For this review, take the finished solid that the model builds, in its own axes (mm). Face numbers are marked on the shaded views. A direction names the side the tool comes from. Round coordinates to 2 decimals unless told otherwise and drop trailing zeros. Order: outer loops, then holes, each group sorted by start corner. A loop starts at its lowest first (then second) coordinate and runs counter-clockwise, first axis right, second up. Notation, with made-up numbers: (10.5, -13.75) - (37.5, -13.75) arc R16 cw to (37.5, -6.75) - close; hole circle Ø9 at (18.25, 84). An arc over 180 degrees is marked (long way). One line per question, with ' | ' between items.
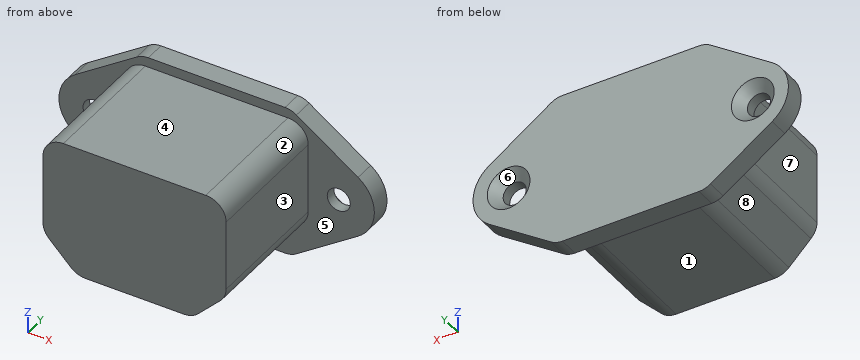
```python
from build123d import *

# Parameters (mm, degrees)
SKIZZE1_W                                    = 27
SKIZZE1_H                                    = 19.5
AUFSATZ_LINEAR_AUSTRAGEN1_DEPTH              = 19.6
FASE1_SIZE                                   = 5
AUFSATZ_LINEAR_AUSTRAGEN2_DEPTH              = 3
VERRUNDUNG1_R                                = 3
FORMSENKUNG_F_R_M3_LINSENSENKSCHRAUB_2_COUNT = 2
FORMSENKUNG_F_R_M3_LINSENSENKSCHRAUB_2_PITCH = 36


with BuildPart() as part:
    # Skizze1 → Aufsatz-Linear austragen1 (new body)
    with BuildSketch(Plane.XY):
        Rectangle(SKIZZE1_W, SKIZZE1_H)
    extrude(amount=AUFSATZ_LINEAR_AUSTRAGEN1_DEPTH)

    # Fase1
    fase1_edges = [part.edges().sort_by_distance(p)[0] for p in [
        (-13.5, 0, 0),
        (13.5, 0, 0),
    ]]
    chamfer(fase1_edges, length=FASE1_SIZE)

    # Skizze2 → Aufsatz-Linear austragen2 (add)
    with BuildSketch(Plane(origin=(0, 9.75, 0), x_dir=(1, 0, 0), z_dir=(0, 1, 0))):
        with BuildLine():
            Line((-11, 1.45), (11, 1.45))
            Line((11, 1.45), (20.845503979, -5.253808724))
            ThreePointArc((20.845503979, -5.253808724), (23.25, -9.8), (20.845503979, -14.346191276))
            Line((20.845503979, -14.346191276), (11, -21.05))
            Line((11, -21.05), (-11, -21.05))
            Line((-11, -21.05), (-20.845503979, -14.346191276))
            ThreePointArc((-20.845503979, -14.346191276), (-23.25, -9.8), (-20.845503979, -5.253808724))
            Line((-20.845503979, -5.253808724), (-11, 1.45))
        make_face()
    extrude(amount=AUFSATZ_LINEAR_AUSTRAGEN2_DEPTH)

    # Verrundung1
    # the kernel refuses this fillet: 3 mm, written as the material it takes off along each edge
    with BuildSketch(Plane(origin=(-13.5, 9.75, 19.6), x_dir=(0, 0, -1), z_dir=(0, -1, 0))) as verrundung1_piece_1:
        with BuildLine():
            CenterArc((VERRUNDUNG1_R, VERRUNDUNG1_R), VERRUNDUNG1_R, 180, 90)
            Line((0, VERRUNDUNG1_R), (0, 0))
            Line((0, 0), (VERRUNDUNG1_R, 0))
        make_face()
    extrude(amount=27, mode=Mode.SUBTRACT)
    with BuildSketch(Plane(origin=(13.5, -12.856601718, 5), x_dir=(0, 0, 1), z_dir=(0, 1, 0)), Plane(origin=(-8.5, 9.75, 0), x_dir=(-0.7071067811865469, 0, 0.707106781186548), z_dir=(0, -1, 0)), Plane(origin=(-13.5, 9.75, 5), x_dir=(0, 0, 1), z_dir=(0, -1, 0))) as verrundung1_piece_2:
        with BuildLine():
            CenterArc((VERRUNDUNG1_R * 0.414213562373, -VERRUNDUNG1_R), VERRUNDUNG1_R, 90, 45)
            Line((-VERRUNDUNG1_R * 0.292893218813, -VERRUNDUNG1_R * 0.292893218813), (0, 0))
            Line((0, 0), (VERRUNDUNG1_R * 0.414213562373, 0))
        make_face()
    extrude(amount=22.606601718, mode=Mode.SUBTRACT)
    with BuildSketch(Plane(origin=(8.5, -12.856601718, 0), x_dir=(-1, 0, 0), z_dir=(0, 1, 0))) as verrundung1_piece_3:
        with BuildLine():
            CenterArc((VERRUNDUNG1_R * 0.414213562373, VERRUNDUNG1_R), VERRUNDUNG1_R, 225, 45)
            Line((-VERRUNDUNG1_R * 0.292893218813, VERRUNDUNG1_R * 0.292893218813), (0, 0))
            Line((0, 0), (VERRUNDUNG1_R * 0.414213562373, 0))
        make_face()
    extrude(amount=22.606601718, mode=Mode.SUBTRACT)
    with BuildSketch(Plane(origin=(11, 7.439046605, -1.45), x_dir=(0.8265802320093436, 0, 0.5628189052007578), z_dir=(0, 1, 0)), Plane(origin=(-11, 7.439046605, -1.45), x_dir=(1, 0, 0), z_dir=(0, 1, 0)), Plane(origin=(-11, 7.439046605, 21.05), x_dir=(-0.8265802320093435, 0, -0.5628189052007582), z_dir=(0, 1, 0))) as verrundung1_piece_4:
        with BuildLine():
            CenterArc((VERRUNDUNG1_R * 0.308127119377, -VERRUNDUNG1_R), VERRUNDUNG1_R, 90, 34.250968868)
            Line((-VERRUNDUNG1_R * 0.254691785823, -VERRUNDUNG1_R * 0.173419767991), (0, 0))
            Line((0, 0), (VERRUNDUNG1_R * 0.308127119377, 0))
        make_face()
    extrude(amount=7.621906791, mode=Mode.SUBTRACT)
    with BuildSketch(Plane(origin=(11, 7.439046605, 21.05), x_dir=(0.8265802320093447, 0, -0.5628189052007564), z_dir=(0, 1, 0))) as verrundung1_piece_5:
        with BuildLine():
            CenterArc((VERRUNDUNG1_R * 0.308127119377, VERRUNDUNG1_R), VERRUNDUNG1_R, 235.749031132, 34.250968868)
            Line((-VERRUNDUNG1_R * 0.254691785823, VERRUNDUNG1_R * 0.173419767991), (0, 0))
            Line((0, 0), (VERRUNDUNG1_R * 0.308127119377, 0))
        make_face()
    extrude(amount=7.621906791, mode=Mode.SUBTRACT)
    with BuildSketch(Plane(origin=(13.5, -17.25, 19.6), x_dir=(-1, 0, 0), z_dir=(0, 1, 0))) as verrundung1_piece_6:
        with BuildLine():
            CenterArc((VERRUNDUNG1_R, -VERRUNDUNG1_R), VERRUNDUNG1_R, 90, 90)
            Line((0, -VERRUNDUNG1_R), (0, 0))
            Line((0, 0), (VERRUNDUNG1_R, 0))
        make_face()
    extrude(amount=27, mode=Mode.SUBTRACT)

    # Skizze4 → Formsenkung für M3 Linsensenkschraube mit Schlitz1 (revolve, cut)
    with BuildSketch(Plane(origin=(-18, 12.75, 9.8), x_dir=(0, 0, 1), z_dir=(1, 0, 0))):
        Polygon((0, 0), (0, 3), (1.7, 3), (1.7, 1.45), (3.15, 0), align=None)
    formsenkung_f_r_m3_linsensenkschraube_mi = revolve(axis=Axis((-18, 19.1, 9.8), (0, -1, 0)), mode=Mode.SUBTRACT)

    # Formsenkung f_r M3 Linsensenkschraub 2: Formsenkung für M3 Linsensenkschraube mit Schlitz1 ×2
    with Locations(*[(i * FORMSENKUNG_F_R_M3_LINSENSENKSCHRAUB_2_PITCH, 0, 0) for i in range(1, FORMSENKUNG_F_R_M3_LINSENSENKSCHRAUB_2_COUNT)]):
        add(formsenkung_f_r_m3_linsensenkschraube_mi, mode=Mode.SUBTRACT)


solid = part.part
```
(1) For probe 1 along X at (y, z) = (10.3, 9.8); probe 2 along X at (y, z) = (4.5, 12); probe 3 along Z at (x, y) = (18, 10.45), list the stretches that pass through material, from the lowest coordinate up. Write a range as [from, to].
Output values:
probe 1: [-23.25, -19.7], [-16.3, 16.3], [19.7, 23.25] | probe 2: [-13.5, 13.5] | probe 3: [3.32, 8.1], [11.5, 16.28]
(2) We need section C-C on y = 7.25. State the section outline as (x, z) points.
Output values:
outline: (-13.5, 6.24) arc R3 ccw to (-12.62, 4.12) - (-9.38, 0.88) arc R3 ccw to (-7.26, 0) - (7.26, 0) arc R3 ccw to (9.38, 0.88) - (12.62, 4.12) arc R3 ccw to (13.5, 6.24) - (13.5, 16.6) arc R3 ccw to (10.5, 19.6) - (-10.5, 19.6) arc R3 ccw to (-13.5, 16.6) - close
(3) We need section A-A on z = 9.8. State the section outline as (x, y) points, plus the area to 3 significant figures.
Output values:
outline: (-23.25, 9.75) - (-19.7, 9.75) - (-19.7, 11.3) - (-21.15, 12.75) - (-23.25, 12.75) - close; (-16.3, 9.75) - (-13.5, 9.75) - (-13.5, -9.75) - (13.5, -9.75) - (13.5, 9.75) - (16.3, 9.75) - (16.3, 11.3) - (14.85, 12.75) - (-14.85, 12.75) - (-16.3, 11.3) - close; (19.7, 9.75) - (23.25, 9.75) - (23.25, 12.75) - (21.15, 12.75) - (19.7, 11.3) - close | area: 641 mm^2
(4) We need section B-B on x = 1. State the section outline as (y, z) points.
Output values:
outline: (-9.75, 0) - (9.75, 0) - (9.75, -1.45) - (12.75, -1.45) - (12.75, 21.05) - (9.75, 21.05) - (9.75, 19.6) - (-9.75, 19.6) - close
(5) Mouldability with a two-part tool opening along Z and no side actions: class the marked faces 6, 7 and 8 as released by +Z, released by -Z, zero draft, split by the parting line, or undercut.
Output values:
face 6: undercut | face 7: zero draft | face 8: released by -Z
(6) We need section D-D on x = 18. State the section outline as (y, z) points.
Output values:
outline: (9.75, 3.32) - (12.75, 3.32) - (12.75, 6.65) - (11.3, 8.1) - (9.75, 8.1) - close; (9.75, 11.5) - (11.3, 11.5) - (12.75, 12.95) - (12.75, 16.28) - (9.75, 16.28) - close
(7) Insertion check: pin 1 (5 mm diameter, centred on y = 1, z = 11, fed in from -X); pin 2 (5.5 mm diameter, centred on x = -18, z = 9.8, fed in from -Y); pin 3 (5 mm diameter, centred on y = 1, z = 11, fed in from +X). Each pin has a flat end and moves straight along its axis. Give the tip position at first contact, or say it passes through.
Output values:
pin 1: x = -13.5 | pin 2: y = 9.75 | pin 3: x = 13.5
(8) For the marked faces 1, 2, 3, 4 and 5, list the 3-axis set-ups (+Z, -Z, +X, -X, +Y, -Y) from which the entire face can be reached by the end or side of a thin tool; tool diameter is ignored.
Output values:
face 1: -Z, +X, -X, -Y | face 2: +Z, +X, -Y | face 3: +Z, -Z, +X, -Y | face 4: +Z, +X, -X, -Y | face 5: -Y
